Part model, mm, in its own coordinate system. Give positions to 0.01 mm unless a question says otherwise; leave off trailing zeros. Loops run counter-clockwise (first coordinate to the right, second up) from the corner with the lowest first, then second, coordinate; pieces in that order, holes last. Notation, with made-up numbers: (25.25, 62) -> (51.25, 62) arc R20 cw to (51.25, 81) -> close; hole circle Ø6 at (-14.75, 76.25). An arc over 180 degrees is marked (long way). One line per question, with ' | ' between items.
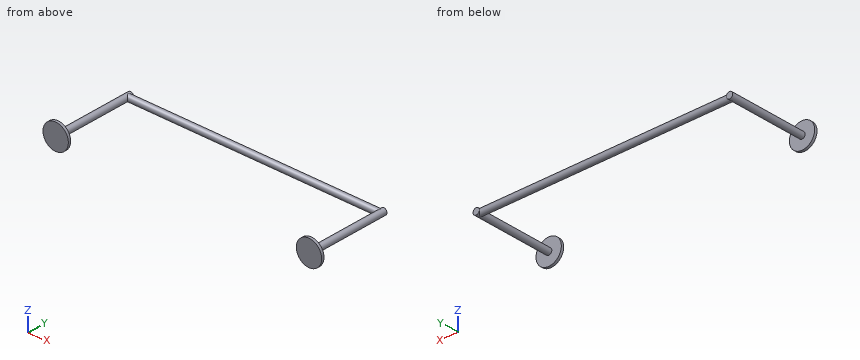
```python
from build123d import *

# Parameters (mm, degrees)
SKETCH_1_R        = 50
EXTRUDE_1_DEPTH   = 10
EXTRUDE_1_2_DEPTH = 10
SKETCH_2_R        = 12.5
EXTRUDE_2_DEPTH   = 315
SKETCH_3_R        = 12.5
EXTRUDE_3_DEPTH   = 1000


with BuildPart() as part:
    # Sketch 1 → Extrude 1 (new body)
    with BuildSketch(Plane(origin=(0, 0, 0), x_dir=(1, 0, 0), z_dir=(0, 1, 0))):
        with Locations(Location((0, 0, 0), (0, 0, 270))):
            Circle(SKETCH_1_R)
    extrude(amount=EXTRUDE_1_DEPTH)



with BuildPart() as body_2:
    # Sketch 1 → Extrude 1 2 (new body)
    with BuildSketch(Plane(origin=(0, 0, 0), x_dir=(1, 0, 0), z_dir=(0, 1, 0))):
        with Locations(Location((1000, 0, 0), (0, 0, 270))):
            Circle(SKETCH_1_R)
    extrude(amount=EXTRUDE_1_2_DEPTH)


with BuildPart() as part_1:
    add(part.part)

    add(body_2.part)  # Extrude 2 merges body 2
    # Sketch 2 → Extrude 2 (add)
    with BuildSketch(Plane(origin=(0, 10, 0), x_dir=(1, 0, 0), z_dir=(0, 1, 0))):
        with Locations(Location((1000, 0, 0), (0, 0, 270))):
            Circle(SKETCH_2_R)
        with Locations(Location((0, 0, 0), (0, 0, 270))):
            Circle(SKETCH_2_R)
    extrude(amount=EXTRUDE_2_DEPTH)


with BuildPart() as extrude_3_tool:
    # Sketch 3 → Extrude 3 (new body)
    with BuildSketch(Plane(origin=(0, 0, 0), x_dir=(0, 0, -1), z_dir=(1, 0, 0))):
        with Locations(Location((0, 311.132818199, 0), (0, 0, 180))):
            Circle(SKETCH_3_R)
    extrude(amount=EXTRUDE_3_DEPTH)


with BuildPart() as part_2:
    add(part_1.part)


with BuildPart() as part_3:
    # Extrude 3: joined with extrude_3_tool
    add(part_2.part.fuse(extrude_3_tool.part, tol=0.00001))


solid = part_3.part
```
1) Saw through at A-A (z = 0). Give the cut face in (x, y), and give its area (3 significant figures).
Found:
outline: (-50, 0) -> (50, 0) -> (50, 10) -> (12.5, 10) -> (12.5, 298.63) -> (987.5, 298.63) -> (987.5, 10) -> (950, 10) -> (950, 0) -> (1050, 0) -> (1050, 10) -> (1012.5, 10) -> (1012.5, 325) -> (987.5, 325) -> (987.5, 323.63) -> (12.5, 323.63) -> (12.5, 325) -> (-12.5, 325) -> (-12.5, 10) -> (-50, 10) -> close | area: 42,100 mm2
2) Pin check, flat tips, straight feed: P1, Ø1, axis at x = 901.5, z = 10, coming from the +Y side; P2, Ø1.5, axis at y = 175, z = -6, coming from the -X side; P3, Ø6, axis at y = 129, z = 4.5, coming from the +X side. Stop position of each tip, or through.
Found:
P1: y = 319.26 | P2: x = -11.34 | P3: x = 1012.41
3) Saw through at C-C (x = 435.5). Give the cut face in (y, z).
Found:
outline: circle Ø25 at (311.13, 0)
4) Saw through at B-B (y = 103). Give the cut face in (x, z), and give its area (3 significant figures).
Found:
outline: circle Ø25 at (0, 0); circle Ø25 at (1000, 0) | area: 982 mm2
5) Drill centre lines: line 1 (X direction, y = 193.5, z = 10); line 2 (Z direction, x = 573.5, y = 312); line 3 (X direction, y = 22.5, z = 6). Where is each one in solid material? Low to high.
Found:
line 1: -7.5 to 7.5, 992.5 to 1007.5 | line 2: -12.47 to 12.47 | line 3: -10.97 to 10.97, 989.03 to 1010.97
